Autodesk Inventor part; units mm, degrees
ref_plane "YZ Plane" through (0, 0, 0) normal (1, 0, 0) x (0, 1, 0)
ref_plane "XZ Plane" through (0, 0, 0) normal (0, 1, 0) x (-1, 0, 0)
ref_plane "XY Plane" through (0, 0, 0) normal (0, 0, 1) x (1, 0, 0)
sketch "Sketch1" plane through (0, 0, 0) normal (0, 0, 1) x (1, 0, 0)
  line L0 (0, 0) -> (0, 19.05)
  line L1 (0, 19.05) -> (0.7937, 19.05)
  line L2 (0.7937, 19.05) -> (0.7938, 0.7937)
  line L3 (0.7938, 0.7937) -> (19.05, 0.7937)
  line L4 (19.05, 0.7937) -> (19.05, 0)
  line L5 (19.05, 0) -> (0, 0)
  dimension "d0" = 19.05
  dimension "d1" = 0.7937
extrude "Extrusion1" add sketch "Sketch1" along normal blind 92.075
sketch "Sketch2" plane through (0, 0, 0) normal (0, -1, 0) x (1, 0, 0)
  line L0 (19.05, 0) -> (0, 0)
  line L1 (19.05, 0) -> (19.05, 92.075)
  line L2 (0, 92.075) -> (19.05, 92.075)
  line L3 (15.875, 92.075) -> (15.875, 0) construction
  circle A0 centre (15.875, 66.675) radius 1.905
  line L4 (9.525, 92.075) -> (9.525, 0) construction
  circle A1 centre (9.525, 12.7) radius 1.905
  dimension "d4" = 3.175
  dimension "d5" = 3.81
  dimension "d6" = 25.4
  dimension "d7" = 12.7
extrude "Extrusion2" cut sketch "Sketch2" against normal through all
sketch "Sketch3" plane through (0, 0, 0) normal (-1, 0, 0) x (0, 0, 1)
  line L0 (0, 0) -> (0, 19.05)
  line L1 (92.075, 19.05) -> (92.075, 0)
  line L2 (0, 9.525) -> (92.075, 9.525) construction
  circle A0 centre (76.2, 9.525) radius 1.5875
  dimension "d10" = 3.175
  dimension "d11" = 15.875
extrude "Extrusion3" cut sketch "Sketch3" against normal through all
properties part number "Hopper Bracing P1" material "Aluminum 6061"
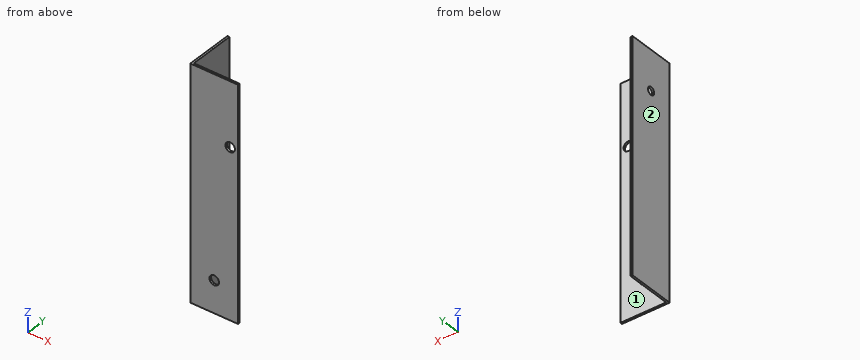
CAD build for the part. Positions are in the model's coordinates, mm. Face numbers are marked on the shaded views. A direction names the side the tool comes from. Coordinates: 2 decimals unless noted, no trailing zeros. Write each loop counter-clockwise with the first axis right and the second up, starting at its lowest first coordinate (ties: lowest second). Pieces come first, ordered by that corner, then holes. Notation, with made-up numbers: M 86.5,13.5 L 92.5,13.5 A22 ccw 92.5,27.5 Z; hole C 23,79 d9. An arc over 180 degrees is marked long. Answer as a JSON object with one key per item and string values. Group by question number.
1) Wall check: line 1 (Y direction, x = 0.2, z = 76.2); line 2 (Y direction, x = 4.5, z = 53). Give the ranges that are in metal, low to high. Write a range as from..to.
2) Saw through at D-D (y = 6). Write the cut outline in (x, z) (3 decimals).
3) Pin check, flat tips, straight feed: pin 1 Ø1 at (x, z) = (9, 56.5) entering from +Y; pin 2 Ø5.5 at (y, z) = (8.5, 50) entering from +X; pin 3 Ø1.9 at (y, z) = (9.525, 76.2) entering from +X. Stop position of each tip, or through.
4) Saw through at A-A (z = 12.7). Write the cut outline in (x, y).
5) Saw through at B-B (x = 15). Write the cut outline in (y, z) (3 decimals).
6) Saw through at C-C (z = 76.2). Write the cut outline in (x, y).
7) Tool access for the marked faces 1 and 2: list every direction of +Z, -Z, +X, -X, +Y, -Y with a clear straight run to the whole face (end or side of a thin tool).
Values follow:
{
 "1": {"line 1": "y = 0..7.94, 11.11..19.05", "line 2": "y = 0..0.79"},
 "2": {"outline": "M 0,0 L 0.794,0 L 0.794,92.075 L 0,92.075 Z"},
 "3": {"pin 1": "stops at y = 0.79", "pin 2": "stops at x = 0.79", "pin 3": "passes through"},
 "4": {"outline": "M 0,0 L 7.62,0 L 7.62,0.79 L 0.79,0.79 L 0.79,19.05 L 0,19.05 Z; M 11.43,0 L 19.05,0 L 19.05,0.79 L 11.43,0.79 Z"},
 "5": {"outline": "M 0,0 L 0.794,0 L 0.794,64.983 L 0,64.983 Z; M 0,68.367 L 0.794,68.367 L 0.794,92.075 L 0,92.075 Z"},
 "6": {"outline": "M 0,0 L 19.05,0 L 19.05,0.79 L 0.79,0.79 L 0.79,7.94 L 0,7.94 Z; M 0,11.11 L 0.79,11.11 L 0.79,19.05 L 0,19.05 Z"},
 "7": {"face 1": "+Z, -Z, +X, +Y", "face 2": "+Z, -Z, -X, +Y, -Y"}
}
